from build123d import *

# Parameters (mm, degrees)
SKETCH_2_R          = 4.8
EXTRUDE_1_DEPTH     = 12
EXTRUDE_2_DEPTH     = 10
SKETCH_4_R          = 5.5
EXTRUDE_3_DEPTH     = 14
SKETCH_5_R          = 4.8
EXTRUDE_4_DEPTH     = 9.5
SKETCH_6_R          = 3.1
CUT_EXTRUDE_1_DEPTH = 46.5


with BuildPart() as part:
    # Эскиз2 → Бобышка-Вытянуть1 (new body)
    with BuildSketch(Plane(origin=(0, 0, 0), x_dir=(1, 0, 0), z_dir=(0, 1, 0))):
        Circle(SKETCH_2_R)
    extrude(amount=EXTRUDE_1_DEPTH)

    # Эскиз3 → Бобышка-Вытянуть2 (add)
    with BuildSketch(Plane(origin=(0, 12, 0), x_dir=(1, 0, 0), z_dir=(0, 1, 0))):
        Polygon((5.0208225, -2.608577151), (4.769505331, 3.043871258), (-0.251317169, 5.652448409), (-5.0208225, 2.608577151), (-4.769505331, -3.043871258), (0.251317169, -5.652448409), align=None)
    extrude(amount=EXTRUDE_2_DEPTH)

    # Эскиз4 → Бобышка-Вытянуть3 (add)
    with BuildSketch(Plane(origin=(0, 22, 0), x_dir=(1, 0, 0), z_dir=(0, 1, 0))):
        Circle(SKETCH_4_R)
    extrude(amount=EXTRUDE_3_DEPTH)

    # Эскиз5 → Бобышка-Вытянуть4 (add)
    with BuildSketch(Plane(origin=(0, 36, 0), x_dir=(1, 0, 0), z_dir=(0, 1, 0))):
        Circle(SKETCH_5_R)
    extrude(amount=EXTRUDE_4_DEPTH)

    # Эскиз6 → Вырез-Вытянуть1 (cut, through all)
    with BuildSketch(Plane(origin=(0, 45.5, 0), x_dir=(1, 0, 0), z_dir=(0, 1, 0))):
        Circle(SKETCH_6_R)
    extrude(amount=-CUT_EXTRUDE_1_DEPTH, mode=Mode.SUBTRACT)


solid = part.part
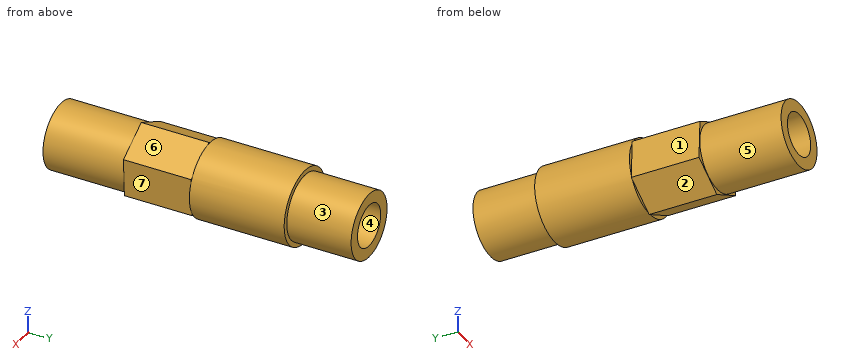
CAD build for the part. Positions are in the model's coordinates, mm. Face numbers are marked on the shaded views. A direction names the side the tool comes from. Round coordinates to 2 decimals unless told otherwise and drop trailing zeros. Order: outer loops, then holes, each group sorted by start corner. A loop starts at its lowest first (then second) coordinate and runs counter-clockwise, first axis right, second up. Notation, with made-up numbers: (9, 42) - (52, 42) arc R12 cw to (52, 56) - close; hole circle Ø6 at (30, -12.75). An arc over 180 degrees is marked (long way). Return JSON: item names as keys, results as strings.
(1) Cut at A-A (x = 2.5). Give the cut face in (y, z), then the cut area to 3 significant figures.
Answer key:
{"outline": "(0, -4.1) - (12, -4.1) - (12, -4.22) - (22, -4.22) - (22, -4.9) - (36, -4.9) - (36, -4.1) - (45.5, -4.1) - (45.5, -1.83) - (0, -1.83) - close; (0, 1.83) - (45.5, 1.83) - (45.5, 4.1) - (36, 4.1) - (36, 4.9) - (22, 4.9) - (22, 4.22) - (12, 4.22) - (12, 4.1) - (0, 4.1) - close", "area": "231 mm^2"}
(2) Pin check, flat tips, straight feed: pin 1 Ø1 at (y, z) = (38.5, -1) entering from +X; pin 2 Ø1.5 at (y, z) = (9, -2.5) entering from -X; pin 3 Ø1.5 at (y, z) = (32.5, -4) entering from +X. Stop position of each tip, or through.
Answer key:
{"pin 1": "stops at x = 4.77", "pin 2": "stops at x = -4.47", "pin 3": "stops at x = 4.44"}
(3) Tool access for the marked faces 1, 2 and 3: list every direction of +Z, -Z, +X, -X, +Y, -Y with a clear straight run to the whole face (end or side of a thin tool).
Answer key:
{"face 1": "+Z, -X, -Y", "face 2": "-Z, -X, -Y", "face 3": "+Y"}
(4) Cut at C-C (y = 31). Give the cut face in (x, z).
Answer key:
{"outline": "circle Ø11 at (0, 0); hole circle Ø6.2 at (0, 0)"}
(5) Wall check: probe 1 along X at (y, z) = (31, 0); probe 2 along X at (y, z) = (11, 0). Give the ranges that are in metal, low to high. Write a range as from..to.
Answer key:
{"probe 1": "x = -5.5..-3.1, 3.1..5.5", "probe 2": "x = -4.8..-3.1, 3.1..4.8"}
(6) Pull direction Z, two halves, no side cores. Call the marked faces 4, 5, 6 and 7: +Z half, -Z half, draft (parallel to the pull), parting line (faces both ways), or undercut.
Answer key:
{"face 4": "undercut", "face 5": "parting line", "face 6": "+Z half", "face 7": "-Z half"}
(7) Cut at B-B (z = -0.5). Give the cut face in (x, y), then the cut area to 3 significant figures.
Answer key:
{"outline": "(-5.48, 22) - (-4.93, 22) - (-4.93, 12) - (-4.77, 12) - (-4.77, 0) - (-3.06, 0) - (-3.06, 45.5) - (-4.77, 45.5) - (-4.77, 36) - (-5.48, 36) - close; (3.06, 0) - (4.77, 0) - (4.77, 12) - (4.88, 12) - (4.88, 22) - (5.48, 22) - (5.48, 36) - (4.77, 36) - (4.77, 45.5) - (3.06, 45.5) - close", "area": "178 mm^2"}
